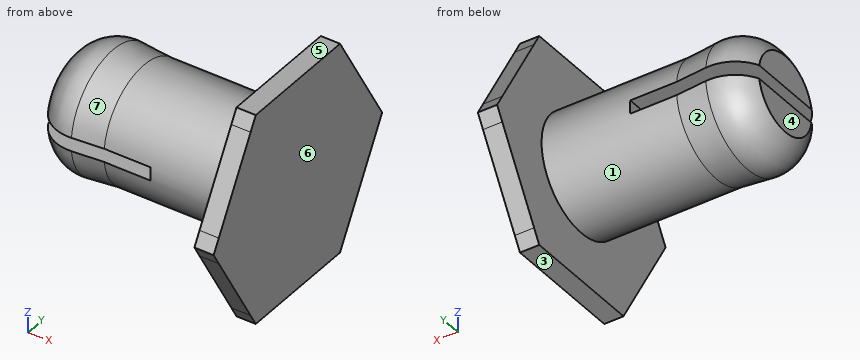
```python
from build123d import *
from build123d import SkipClean  # not in build123d's __all__

# Parameters (mm, degrees)
F3_DEPTH = 6
F4_W     = 13.7017059222
F4_H     = 13
F4_R     = 3
F5_DEPTH = 25
F6_DEPTH = 1


with BuildPart() as f1:
    # F0 (on Front) → F1 (revolve)
    with BuildSketch(Plane.XZ):
        with BuildLine():
            Line((-11.5940445242, 0), (0, 0))
            Line((0, 0), (0, 6))
            Line((0, 6), (-1, 6))
            Line((-1, 6), (-1, 3))
            Line((-1, 3), (-8, 3))
            Line((-8, 3), (-9.6100640914, 3.1408623555))
            ThreePointArc((-9.6100640914, 3.1408623555), (-10.7813661664, 2.8822577685), (-11.5940445242, 2))
            Line((-11.5940445242, 2), (-11.5940445242, 0))
        make_face()
    revolve(axis=Axis((-5.7970222621, 0, 0), (1, 0, 0)))

    # F2 (on face) → F3 (cut)
    with BuildSketch(Plane(origin=(-11.5940445242, 0, 0), x_dir=(0, -1, 0), z_dir=(-1, 0, 0))):
        with BuildLine():
            ThreePointArc((-1.9691368668, -0.35), (-2, 0), (-1.9691368668, 0.35))
            Line((-1.9691368668, 0.35), (-4, 0.35))
            Line((-4, 0.35), (-4, -0.35))
            Line((-4, -0.35), (-2.9795133831, -0.35))
            Line((-2.9795133831, -0.35), (-1.9691368668, -0.35))
        make_face()
        with BuildLine():
            Line((1.9691368668, 0.35), (0.25, 0.35))
            Line((0.25, 0.35), (0.25, 0))
            Line((0.25, 0), (0.25, -0.35))
            Line((0.25, -0.35), (1.9691368668, -0.35))
            ThreePointArc((1.9691368668, -0.35), (1.9922692757, -0.1756790632), (2, 0))
            ThreePointArc((2, 0), (1.9922692757, 0.1756790632), (1.9691368668, 0.35))
        make_face()
        with BuildLine():
            Line((-0.25, 0), (-0.25, 0.35))
            Line((-0.25, 0.35), (-1.9691368668, 0.35))
            ThreePointArc((-1.9691368668, 0.35), (-2, 0), (-1.9691368668, -0.35))
            Line((-1.9691368668, -0.35), (-0.25, -0.35))
            Line((-0.25, -0.35), (-0.25, 0))
        make_face()
        Polygon((0.25, 0), (0.25, 0.35), (-0.25, 0.35), (-0.25, 0), (-0.25, -0.35), (0.25, -0.35), align=None)
        with BuildLine():
            Line((4, 0.35), (1.9691368668, 0.35))
            ThreePointArc((1.9691368668, 0.35), (1.9922692757, 0.1756790632), (2, 0))
            ThreePointArc((2, 0), (1.9922692757, -0.1756790632), (1.9691368668, -0.35))
            Line((1.9691368668, -0.35), (2.9795133831, -0.35))
            Line((2.9795133831, -0.35), (4, -0.35))
            Line((4, -0.35), (4, 0.35))
        make_face()
    extrude(amount=-F3_DEPTH, mode=Mode.SUBTRACT)

    # F4 (on face) → F5 (cut)
    with BuildSketch(Plane(origin=(-1, 0, 0), x_dir=(0, -1, 0), z_dir=(-1, 0, 0))):
        Rectangle(F4_W, F4_H)
        Polygon((-6.3508529611, 0), (-3.1754264805, 5.5), (3.1754264805, 5.5), (6.3508529611, 0), (3.1754264805, -5.5), (-3.1754264805, -5.5), align=None, mode=Mode.SUBTRACT)
        with BuildLine():
            Line((2.3979157617, 5.5), (-2.3979157617, 5.5))
            ThreePointArc((-2.3979157617, 5.5), (-3, 5.1961524227), (-3.56418184, 4.8266559657))
            Line((-3.56418184, 4.8266559657), (-5.9620976016, 0.6733440343))
            ThreePointArc((-5.9620976016, 0.6733440343), (-6, 0), (-5.9620976016, -0.6733440343))
            Line((-5.9620976016, -0.6733440343), (-3.56418184, -4.8266559657))
            ThreePointArc((-3.56418184, -4.8266559657), (-3, -5.1961524227), (-2.3979157617, -5.5))
            Line((-2.3979157617, -5.5), (2.3979157617, -5.5))
            ThreePointArc((2.3979157617, -5.5), (3, -5.1961524227), (3.56418184, -4.8266559657))
            Line((3.56418184, -4.8266559657), (5.9620976016, -0.6733440343))
            ThreePointArc((5.9620976016, -0.6733440343), (5.9905169063, -0.3372049749), (6, 0))
            ThreePointArc((6, 0), (5.9905169063, 0.3372049749), (5.9620976016, 0.6733440343))
            Line((5.9620976016, 0.6733440343), (3.56418184, 4.8266559657))
            ThreePointArc((3.56418184, 4.8266559657), (3, 5.1961524227), (2.3979157617, 5.5))
        make_face()
        Circle(F4_R, mode=Mode.SUBTRACT)
    with SkipClean():  # cleaning this boolean's faces spoils the solid; the shape is the same uncleaned
        extrude(amount=-F5_DEPTH, mode=Mode.SUBTRACT)

    # F4 (on face) → F6 (join)
    with BuildSketch(Plane(origin=(-1, 0, 0), x_dir=(0, -1, 0), z_dir=(-1, 0, 0))):
        with BuildLine():
            Line((2.3979157617, 5.5), (-2.3979157617, 5.5))
            ThreePointArc((-2.3979157617, 5.5), (-3, 5.1961524227), (-3.56418184, 4.8266559657))
            Line((-3.56418184, 4.8266559657), (-5.9620976016, 0.6733440343))
            ThreePointArc((-5.9620976016, 0.6733440343), (-6, 0), (-5.9620976016, -0.6733440343))
            Line((-5.9620976016, -0.6733440343), (-3.56418184, -4.8266559657))
            ThreePointArc((-3.56418184, -4.8266559657), (-3, -5.1961524227), (-2.3979157617, -5.5))
            Line((-2.3979157617, -5.5), (2.3979157617, -5.5))
            ThreePointArc((2.3979157617, -5.5), (3, -5.1961524227), (3.56418184, -4.8266559657))
            Line((3.56418184, -4.8266559657), (5.9620976016, -0.6733440343))
            ThreePointArc((5.9620976016, -0.6733440343), (5.9905169063, -0.3372049749), (6, 0))
            ThreePointArc((6, 0), (5.9905169063, 0.3372049749), (5.9620976016, 0.6733440343))
            Line((5.9620976016, 0.6733440343), (3.56418184, 4.8266559657))
            ThreePointArc((3.56418184, 4.8266559657), (3, 5.1961524227), (2.3979157617, 5.5))
        make_face()
        Circle(F4_R, mode=Mode.SUBTRACT)
        with BuildLine():
            Line((-2.3979157617, 5.5), (-3.1754264805, 5.5))
            Line((-3.1754264805, 5.5), (-3.56418184, 4.8266559657))
            ThreePointArc((-3.56418184, 4.8266559657), (-3, 5.1961524227), (-2.3979157617, 5.5))
        make_face()
        with BuildLine():
            Line((3.1754264805, 5.5), (2.3979157617, 5.5))
            ThreePointArc((2.3979157617, 5.5), (3, 5.1961524227), (3.56418184, 4.8266559657))
            Line((3.56418184, 4.8266559657), (3.1754264805, 5.5))
        make_face()
        with BuildLine():
            Line((6.3508529611, 0), (5.9620976016, 0.6733440343))
            ThreePointArc((5.9620976016, 0.6733440343), (5.9905169063, 0.3372049749), (6, 0))
            ThreePointArc((6, 0), (5.9905169063, -0.3372049749), (5.9620976016, -0.6733440343))
            Line((5.9620976016, -0.6733440343), (6.3508529611, 0))
        make_face()
        with BuildLine():
            ThreePointArc((3.56418184, -4.8266559657), (3, -5.1961524227), (2.3979157617, -5.5))
            Line((2.3979157617, -5.5), (3.1754264805, -5.5))
            Line((3.1754264805, -5.5), (3.56418184, -4.8266559657))
        make_face()
        with BuildLine():
            ThreePointArc((-2.3979157617, -5.5), (-3, -5.1961524227), (-3.56418184, -4.8266559657))
            Line((-3.56418184, -4.8266559657), (-3.1754264805, -5.5))
            Line((-3.1754264805, -5.5), (-2.3979157617, -5.5))
        make_face()
        with BuildLine():
            ThreePointArc((-5.9620976016, -0.6733440343), (-6, 0), (-5.9620976016, 0.6733440343))
            Line((-5.9620976016, 0.6733440343), (-6.3508529611, 0))
            Line((-6.3508529611, 0), (-5.9620976016, -0.6733440343))
        make_face()
    extrude(amount=-F6_DEPTH)


solid = f1.part
```
Model file for the job. Use its own axes, mm. Face numbers are marked on the shaded views. A direction names the side the tool comes from. Coordinates: 2 decimals unless noted, no trailing zeros. Order: outer loops, then holes, each group sorted by start corner. A loop starts at its lowest first (then second) coordinate and runs counter-clockwise, first axis right, second up. Notation, with made-up numbers: (24.25, 31.25) - (33.25, 31.25) arc R24 cw to (33.25, 45.25) - close; hole circle Ø7 at (-22.75, -9.75). An arc over 180 degrees is marked (long way). Return JSON: item names as keys, results as strings. Group by question number.
1) Flat gauge pins, fed straight in: P1, Ø3, axis at x = -8.5, y = -1, coming from the +Z side; P2, Ø0.6, axis at y = -1, z = 0, coming from the -X side; P3, Ø3, axis at x = -1.5, y = 5, coming from the +Z side. Where does each tip first touch, or does it go through?
2) Saw through at C-C, the plane z = 3.75. Write the cut outline in (x, y).
3) Tool access for the marked faces 1, 2 and 3: list every direction of +Z, -Z, +X, -X, +Y, -Y with a clear straight run to the whole face (end or side of a thin tool).
4) Probe line 1 (X direction, y = 1, z = -5); line 2 (Z direction, x = -10.5, y = -1.5); line 3 (X direction, y = -2.5, z = 0). List the from-to ranges inside material, lowest first. Write a range as from..to.
5) Mould opens along X. For the marked faces 4, 5, 6 and 7 say: released by +X, released by -X, zero draft, split by the parting line, or undercut.
6) Saw through at D-D, the plane y = -5.5. Write the cut outline in (x, z).
7) Saw through at B-B, the plane x = -2.25. Write the cut outline in (y, z), plus the area to 3 significant figures.
8) Saw through at A-A, the plane x = -9. Write the cut outline in (y, z), plus the area to 3 significant figures.
Values found:
{
 "1": {"P1": "stops at z = 3.15", "P2": "stops at x = -5.59", "P3": "stops at z = 4.79"},
 "2": {"outline": "(-1, -4.19) - (0, -4.19) - (0, 4.19) - (-1, 4.19) - close"},
 "3": {"face 1": "none", "face 2": "-Z", "face 3": "-Z, +X, -X, +Y, -Y"},
 "4": {"line 1": "x = -1..0", "line 2": "z = -2.62..-0.35, 0.35..2.62", "line 3": "x = -5.59..0"},
 "5": {"face 4": "released by -X", "face 5": "zero draft", "face 6": "released by +X", "face 7": "undercut"},
 "6": {"outline": "(-1, -1.47) - (0, -1.47) - (0, 1.47) - (-1, 1.47) - close"},
 "7": {"outline": "circle Ø6 at (0, 0)", "area": "28.3 mm²"},
 "8": {"outline": "(-3.07, -0.35) arc R3.09 ccw to (3.07, -0.35) - close; (-3.07, 0.35) - (3.07, 0.35) arc R3.09 ccw to start", "area": "25.6 mm²"}
}
